```python
from build123d import *

# Parameters (mm, degrees)
BOSS_EXTRUDE1_DEPTH = 12.7
CUT_EXTRUDE1_REACH  = 220.591
SKETCH3_R           = 3.175
CUT_EXTRUDE2_DEPTH  = 213.321819416


with BuildPart() as part:
    # Sketch1 → Boss-Extrude1 (new body)
    with BuildSketch(Plane.XY):
        Polygon((-215.9, 0), (215.9, 0), (215.9, -31.75), (132.08, -31.75), (127, -26.67), (-127, -26.67), (-132.08, -31.75), (-215.9, -31.75), align=None)
    extrude(amount=BOSS_EXTRUDE1_DEPTH)

    # Sketch2 → Cut-Extrude1 (cut, up to next)
    with BuildSketch(Plane(origin=(0, 0, 0), x_dir=(1, 0, 0), z_dir=(0, 1, 0)), mode=Mode.PRIVATE) as cut_extrude1_sk1:
        with BuildLine():
            Line((-209.55, 0), (-215.9, 0))
            Line((-215.9, 0), (-215.9, -12.7))
            Line((-215.9, -12.7), (-209.55, -12.7))
            ThreePointArc((-209.55, -12.7), (-208.743444248, -6.35), (-209.55, 0))
        make_face()
    cut_extrude1_tool1 = extrude(cut_extrude1_sk1.sketch, amount=-CUT_EXTRUDE1_REACH, mode=Mode.PRIVATE) & part.part
    cut_extrude1 = cut_extrude1_tool1.solids().sort_by_distance((-212.451105, 0, 6.35))[0]
    add(cut_extrude1, mode=Mode.SUBTRACT)

    # Mirror1: Cut-Extrude1 across plane
    add(cut_extrude1.mirror(Plane(origin=(0, 0, 0), x_dir=(0, 0, 1), z_dir=(1, 0, 0))), mode=Mode.SUBTRACT)

    # Sketch3 → Cut-Extrude2 (cut, through all)
    with BuildSketch(Plane.XY.offset(12.7)):
        with Locations((-199.39, -15.24)):
            Circle(SKETCH3_R)
        with Locations((-187.96, -15.24)):
            Circle(SKETCH3_R)
        with Locations((-176.53, -15.24)):
            Circle(SKETCH3_R)
        with Locations((-165.1, -15.24)):
            Circle(SKETCH3_R)
        with Locations((-153.67, -15.24)):
            Circle(SKETCH3_R)
        with Locations((-142.24, -15.24)):
            Circle(SKETCH3_R)
        with Locations((-130.81, -15.24)):
            Circle(SKETCH3_R)
        with Locations((-119.38, -15.24)):
            Circle(SKETCH3_R)
        with Locations((-107.95, -15.24)):
            Circle(SKETCH3_R)
        with Locations((-96.52, -15.24)):
            Circle(SKETCH3_R)
        with Locations((-85.09, -15.24)):
            Circle(SKETCH3_R)
        with Locations((-73.66, -15.24)):
            Circle(SKETCH3_R)
        with Locations((-62.23, -15.24)):
            Circle(SKETCH3_R)
        with Locations((-50.8, -15.24)):
            Circle(SKETCH3_R)
        with Locations((-39.37, -15.24)):
            Circle(SKETCH3_R)
        with Locations((-27.94, -15.24)):
            Circle(SKETCH3_R)
        with Locations((-16.51, -15.24)):
            Circle(SKETCH3_R)
        with Locations((-5.08, -15.24)):
            Circle(SKETCH3_R)
        with Locations((6.35, -15.24)):
            Circle(SKETCH3_R)
        with Locations((17.78, -15.24)):
            Circle(SKETCH3_R)
        with Locations((29.21, -15.24)):
            Circle(SKETCH3_R)
        with Locations((40.64, -15.24)):
            Circle(SKETCH3_R)
        with Locations((52.07, -15.24)):
            Circle(SKETCH3_R)
        with Locations((63.5, -15.24)):
            Circle(SKETCH3_R)
        with Locations((74.93, -15.24)):
            Circle(SKETCH3_R)
        with Locations((86.36, -15.24)):
            Circle(SKETCH3_R)
        with Locations((97.79, -15.24)):
            Circle(SKETCH3_R)
        with Locations((109.22, -15.24)):
            Circle(SKETCH3_R)
        with Locations((120.65, -15.24)):
            Circle(SKETCH3_R)
        with Locations((132.08, -15.24)):
            Circle(SKETCH3_R)
        with Locations((143.51, -15.24)):
            Circle(SKETCH3_R)
        with Locations((154.94, -15.24)):
            Circle(SKETCH3_R)
        with Locations((166.37, -15.24)):
            Circle(SKETCH3_R)
        with Locations((177.8, -15.24)):
            Circle(SKETCH3_R)
        with Locations((189.23, -15.24)):
            Circle(SKETCH3_R)
        with Locations((200.66, -15.24)):
            Circle(SKETCH3_R)
    extrude(amount=-CUT_EXTRUDE2_DEPTH, mode=Mode.SUBTRACT)


solid = part.part
```
The listing builds one solid part. Answer for the finished solid, in the listing's coordinates (mm). Coordinates: 2 decimals unless noted, no trailing zeros. Write each question's results on one line, items separated by ' | '. Start each with the question number.
1) A cutting plane is placed at A-A (z = 8.25). Count the separate pieces of the cut face and the enclosed holes in it, then the cut area to 3 significant figures.
2) For a pull along X with two mould halves and no side action, classify faces 1 (the cylindrical face through (208.744, -15.653, 6.44)), 2 (the flat face through (-170, -31.75, 6)), 3 (the cylindrical face through (180.73, -16.46, 6.44)) as +X half, -X half, draft (parallel to the pull), parting line (faces both ways), or undercut.
3) Flat-ended cylindrical pins translate along their axes: pin 1 Ø4 at (x, y) = (-5.08, -15.24) entering from +Z; pin 2 Ø7.5 at (x, y) = (6.35, -15.24) entering from +Z; pin 3 Ø3 at (y, z) = (-5.5, 8.5) entering from +X. Find the tip coordinate at first contact, or state that the pin passes through.
4) Straight lines are drawn through the part: probe 1 along Y at (x, z) = (-85.09, 7.25) (3 decimals); probe 2 along Y at (x, z) = (143.51, 4) (3 decimals); probe 3 along X at (y, z) = (-21, 7). For each, find the intervals that lie inside material, in ascending order.
Values follow:
1) separate pieces: 1 | enclosed holes: 36 | area: 10,800 mm²
2) face 1: +X half | face 2: draft | face 3: undercut
3) pin 1: through | pin 2: z = 12.7 | pin 3: x = 209.01
4) probe 1: -26.67 to -18.415, -12.065 to 0 | probe 2: -31.75 to -18.415, -12.065 to 0 | probe 3: -208.75 to 208.75
